Model file for the job. Use its own axes, mm. A direction names the side the tool comes from. Coordinates: 2 decimals unless noted, no trailing zeros. Loops run counter-clockwise (first coordinate to the right, second up) from the corner with the lowest first, then second, coordinate; pieces in that order, holes last. Notation, with made-up numbers: (-29.75, 59) - (22.25, 59) arc R13 cw to (22.25, 68) - close; hole circle Ø11 at (11, 34.25). An arc over 180 degrees is marked (long way). Write each question's results on one line, items separated by ' | '. Start each with the question number.
```python
from build123d import *

# Parameters (mm, degrees)
SKETCH2_W           = 24.690663142
SKETCH2_H           = 2.894566797
BOSS_EXTRUDE2_DEPTH = 5
SKETCH2_2_W         = 24.690663142
SKETCH2_2_H         = 2.894566797
BOSS_EXTRUDE3_DEPTH = 2
SKETCH8_W           = 2.5
SKETCH8_H           = 7
BOSS_EXTRUDE4_DEPTH = 5.96
SKETCH10_W          = 7
SKETCH10_H          = 2.49
BOSS_EXTRUDE5_DEPTH = 3
SKETCH11_W          = 7
SKETCH11_H          = 2.49
BOSS_EXTRUDE6_DEPTH = 5
SKETCH12_W          = 17
SKETCH12_H          = 2.5
BOSS_EXTRUDE7_DEPTH = 10
CUT_EXTRUDE7_REACH  = 37.323
SKETCH14_W          = 13
SKETCH14_H          = 8.75
SKETCH16_W          = 17
SKETCH16_H          = 1.25
BOSS_EXTRUDE8_DEPTH = 9.5
CUT_EXTRUDE8_REACH  = 28.801
SKETCH17_R          = 3.51
FILLET7_R           = 2
FILLET8_R           = 5
FILLET9_R           = 5
CHAMFER1_SIZE       = 2
CHAMFER2_SIZE       = 2
FILLET11_R          = 2
FILLET12_R          = 2
FILLET13_R          = 2
FILLET14_R          = 2
FILLET16_R          = 2
CHAMFER3_SIZE       = 0.5


with BuildPart() as part:
    # Sketch2 → Boss-Extrude2 (new body)
    with BuildSketch(Plane.XY):
        with Locations((0, 20.897290887)):
            Rectangle(SKETCH2_W, SKETCH2_H)
    extrude(amount=BOSS_EXTRUDE2_DEPTH)

    # Sketch2_2 → Boss-Extrude3 (add)
    with BuildSketch(Plane.XY):
        with Locations((0, 20.897290887)):
            Rectangle(SKETCH2_2_W, SKETCH2_2_H)
    extrude(amount=-BOSS_EXTRUDE3_DEPTH)

    # Sketch8 → Boss-Extrude4 (add)
    with BuildSketch(Plane(origin=(0, 19.450007488, 0), x_dir=(-1, 0, 0), z_dir=(0, -1, 0))):
        with Locations((11.1, -1.5)):
            Rectangle(SKETCH8_W, SKETCH8_H)
        with Locations((-11.1, -1.5)):
            Rectangle(SKETCH8_W, SKETCH8_H)
    extrude(amount=BOSS_EXTRUDE4_DEPTH)

    # Sketch10 → Boss-Extrude5 (add)
    with BuildSketch(Plane.ZY.offset(-9.85)):
        with Locations((1.5, 14.735007488)):
            Rectangle(SKETCH10_W, SKETCH10_H)
    extrude(amount=BOSS_EXTRUDE5_DEPTH)

    # Sketch11 → Boss-Extrude6 (add)
    with BuildSketch(Plane(origin=(-9.85, 0, 0), x_dir=(0, 0, -1), z_dir=(1, 0, 0))):
        with Locations((-1.5, 14.735007488)):
            Rectangle(SKETCH11_W, SKETCH11_H)
    extrude(amount=BOSS_EXTRUDE6_DEPTH)

    # Sketch12 → Boss-Extrude7 (add)
    with BuildSketch(Plane(origin=(0, 22.344574285, 0), x_dir=(1, 0, 0), z_dir=(0, 1, 0))):
        with Locations((0, -3.75)):
            Rectangle(SKETCH12_W, SKETCH12_H)
    extrude(amount=BOSS_EXTRUDE7_DEPTH)

    # Sketch14 → Cut-Extrude7 (cut, up to next)
    with BuildSketch(Plane.XY.offset(5), mode=Mode.PRIVATE) as cut_extrude7_sk1:
        with Locations((0, 26.719574285)):
            Rectangle(SKETCH14_W, SKETCH14_H)
    cut_extrude7_tool1 = extrude(cut_extrude7_sk1.sketch, amount=-CUT_EXTRUDE7_REACH, mode=Mode.PRIVATE) & part.part
    add(cut_extrude7_tool1.solids().sort_by_distance((0, 26.719574, 5))[0], mode=Mode.SUBTRACT)

    # Sketch16 → Boss-Extrude8 (add)
    with BuildSketch(Plane.XY.offset(5)):
        with Locations((0, 31.719574285)):
            Rectangle(SKETCH16_W, SKETCH16_H)
    extrude(amount=BOSS_EXTRUDE8_DEPTH)

    # Sketch17 → Cut-Extrude8 (cut, up to next)
    with BuildSketch(Plane(origin=(0, 32.344574285, 0), x_dir=(1, 0, 0), z_dir=(0, 1, 0)), mode=Mode.PRIVATE) as cut_extrude8_sk1:
        with Locations(Location((0, -9, 0), (0, 0, 270))):
            Circle(SKETCH17_R)
    cut_extrude8_tool1 = extrude(cut_extrude8_sk1.sketch, amount=-CUT_EXTRUDE8_REACH, mode=Mode.PRIVATE) & part.part
    add(cut_extrude8_tool1.solids().sort_by_distance((0, 32.344574, 9))[0], mode=Mode.SUBTRACT)

    # Fillet7
    fillet7_edges = [part.edges().sort_by_distance(p)[0] for p in [
        (7.5, 31.094574285, 5),
    ]]
    fillet(fillet7_edges, radius=FILLET7_R)

    # Fillet8
    fillet8_edges = [part.edges().sort_by_distance(p)[0] for p in [
        (8.5, 31.719574285, 14.5),
    ]]
    fillet(fillet8_edges, radius=FILLET8_R)

    # Fillet9
    fillet9_edges = [part.edges().sort_by_distance(p)[0] for p in [
        (-8.5, 31.719574285, 14.5),
    ]]
    fillet(fillet9_edges, radius=FILLET9_R)

    # Chamfer1
    chamfer1_edges = [part.edges().sort_by_distance(p)[0] for p in [
        (-12.35, 13.490007488, 1.5),
    ]]
    chamfer(chamfer1_edges, length=CHAMFER1_SIZE)

    # Chamfer2
    chamfer2_edges = [part.edges().sort_by_distance(p)[0] for p in [
        (12.35, 13.490007488, 1.5),
    ]]
    chamfer(chamfer2_edges, length=CHAMFER2_SIZE)

    # Fillet11
    fillet11_edges = [part.edges().sort_by_distance(p)[0] for p in [
        (-8.5, 22.344574285, 3.75),
    ]]
    fillet(fillet11_edges, radius=FILLET11_R)

    # Fillet12
    fillet12_edges = [part.edges().sort_by_distance(p)[0] for p in [
        (8.5, 22.344574285, 3.75),
    ]]
    fillet(fillet12_edges, radius=FILLET12_R)

    # Fillet13
    fillet13_edges = [part.edges().sort_by_distance(p)[0] for p in [
        (8.5, 22.344574285, 2.5),
    ]]
    fillet(fillet13_edges, radius=FILLET13_R)

    # Fillet14
    fillet14_edges = [part.edges().sort_by_distance(p)[0] for p in [
        (-8.5, 22.344574285, 2.5),
    ]]
    fillet(fillet14_edges, radius=FILLET14_R)

    # Fillet16
    fillet16_edges = [part.edges().sort_by_distance(p)[0] for p in [
        (-7.5, 31.094574285, 5),
    ]]
    fillet(fillet16_edges, radius=FILLET16_R)

    # Chamfer3
    chamfer3_edges = [part.edges().sort_by_distance(p)[0] for p in [
        (0, 32.344574285, 5.49),
    ]]
    chamfer(chamfer3_edges, length=CHAMFER3_SIZE)


solid = part.part
```
Q1. Cut at A-A (y = 15). List the corners of the cut face in (x, z), and give its area (3 significant figures).
Q2. Cut at B-B (z = 9). List the corners of the cut face in (x, y), and give its area (3 significant figures).
Q3. Cut at D-D (x = 0). List the corners of the cut face in (y, z).
Q4. Mould opens along Y. For faces 5 (the cylindrical face through (-7, 31.73, 13.07)), 6 (the flat face through (-7, 15.98, 2)), 7 (the flat face through (-11.34, 14.48, 1.55)) say: +Y half, -Y half, draft (parallel to the pull), parting line (faces both ways), or undercut.
Q5. Pin check, flat tips, straight feed: pin 1 (2 mm diameter, centred on x = 8, z = 8.5, fed in from -Y); pin 2 (5 mm diameter, centred on y = 27.5, z = 4, fed in from -X); pin 3 (5 mm diameter, centred on y = 27.5, z = 5, fed in from +X). Stop position of each tip, or through.
Q6. Which spindle directions (+Z, -Z, +X, -X, +Y, -Y) get a long thin tool onto all of the face, cutting with end or side? Do faces 1 (the flat face through (1.8, 31.095, 5.7)), 2 (the flat face through (6.85, 15, 1)), 3 (the flat face through (-6.5, 27, 4)), 4 (the flat face through (8.5, 29, 4)). Say none if no direction does.
Q7. Cut at C-C (x = -7.5). List the corners of the cut face in (y, z).
Q8. Drill centre lines: L1, parallel to X at y = 31.7, z = 9; L2, parallel to Y at x = -5, z = 1.25; L3, parallel to Y at x = 4.5, z = 4.5. Where is each one in solid material? Low to high. Write a range as from..to.
Check result:
1) outline: (-11.86, -2) - (-4.85, -2) - (-4.85, 5) - (-11.86, 5) - close; (6.85, -2) - (11.86, -2) - (11.86, 5) - (6.85, 5) - close | area: 84.1 mm²
2) outline: (-8.5, 31.09) - (-3.51, 31.09) - (-3.51, 31.84) - (-4.01, 32.34) - (-8.5, 32.34) - close; (3.51, 31.09) - (8.5, 31.09) - (8.5, 32.34) - (4.01, 32.34) - (3.51, 31.84) - close | area: 12.2 mm²
3) outline: (19.45, -2) - (22.34, -2) - (22.34, 5) - (19.45, 5) - close; (31.09, 2.5) - (32.34, 2.5) - (32.34, 4.99) - (31.84, 5.49) - (31.09, 5.49) - close; (31.09, 12.51) - (31.84, 12.51) - (32.34, 13.01) - (32.34, 14.5) - (31.09, 14.5) - close
4) face 5: draft | face 6: undercut | face 7: -Y half
5) pin 1: y = 31.09 | pin 2: x = -8.5 | pin 3: x = 8.5
6) face 1: +Z | face 2: +Z, -Z, -Y | face 3: +Z, -Z | face 4: +Z, -Z, +X, +Y
7) outline: (13.49, -2) - (15.98, -2) - (15.98, 5) - (13.49, 5) - close; (19.45, -2) - (22.34, -2) - (22.34, 0.5) arc R2 cw to (24.34, 2.5) - (32.34, 2.5) - (32.34, 12.5) - (31.09, 12.5) - (31.09, 7) arc R2 cw to (29.09, 5) - (19.45, 5) - close
8) L1: -8.5..-3.51, 3.51..8.5 | L2: 13.49..15.98, 19.45..22.34 | L3: 19.45..22.34, 31.09..32.34
